Here's how the part is built. I have some questions about the finished solid (model axes, mm). A direction names the side the tool comes from. Round coordinates to 2 decimals unless told otherwise and drop trailing zeros. Write each loop counter-clockwise with the first axis right and the second up, starting at its lowest first coordinate (ties: lowest second). Pieces come first, ordered by that corner, then holes. Notation, with made-up numbers: (41, 2) -> (80, 2) arc R12 cw to (80, 16) -> close; hole circle Ø10 at (89, 87). An arc over 180 degrees is marked (long way). Answer in a Markdown table with one row per item. Add a question column.
from build123d import *

# Parameters (mm, degrees)
BOSS_EXTRU_1_DEPTH      = 23
BOSS_EXTRU_2_DEPTH      = 3
ENL_V_MAT_EXTRU_1_DEPTH = 3
ESQUISSE4_R             = 2.6
ENL_V_MAT_EXTRU_2_DEPTH = 3
ESQUISSE5_R             = 2.6
ENL_V_MAT_EXTRU_3_DEPTH = 3
ESQUISSE6_R             = 2.6
ENL_V_MAT_EXTRU_4_DEPTH = 3
CONG_1_R                = 10


with BuildPart() as part:
    # Esquisse1 → Boss.-Extru.1 (new body)
    with BuildSketch(Plane.XY):
        Polygon((100, 92.65), (100, 112.65), (97, 112.65), (97, 93.123594611), (90.984838829, 74.546771861), (93.838946748, 73.622613873), align=None)
    extrude(amount=BOSS_EXTRU_1_DEPTH)

    # Esquisse2 → Boss.-Extru.2 (add)
    with BuildSketch(Plane.XY):
        Polygon((90.984838829, 74.546771861), (79, 74.546771861), (79, 112.65), (97, 112.65), (97, 93.123594611), align=None)
    extrude(amount=BOSS_EXTRU_2_DEPTH)

    # Esquisse3 → Enlèv. mat.-Extru.1 (cut)
    with BuildSketch(Plane.XY.offset(3)):
        Polygon((90.984838829, 74.546771861), (79, 78.427453619), (79, 74.546771861), align=None)
    extrude(amount=-ENL_V_MAT_EXTRU_1_DEPTH, mode=Mode.SUBTRACT)

    # Esquisse4 → Enlèv. mat.-Extru.2 (cut)
    with BuildSketch(Plane.XY.offset(3)):
        with Locations((88, 102.65)):
            Circle(ESQUISSE4_R)
        with Locations((88, 82.65)):
            Circle(ESQUISSE4_R)
    extrude(amount=-ENL_V_MAT_EXTRU_2_DEPTH, mode=Mode.SUBTRACT)

    # Esquisse5 → Enlèv. mat.-Extru.3 (cut)
    with BuildSketch(Plane.ZY.offset(-97)):
        with Locations((13, 102.886797306)):
            Circle(ESQUISSE5_R)
    extrude(amount=-ENL_V_MAT_EXTRU_3_DEPTH, mode=Mode.SUBTRACT)

    # Esquisse6 → Enlèv. mat.-Extru.4 (cut)
    with BuildSketch(Plane(origin=(60.503141075, -19.590871368, 0), x_dir=(0, 0, 1), z_dir=(-0.9513693063481516, 0.30805266260598485, 0))):
        with Locations(Location((13, 108.712835188, 0), (0, 0, 270))):
            Circle(ESQUISSE6_R)
    extrude(amount=-ENL_V_MAT_EXTRU_4_DEPTH, mode=Mode.SUBTRACT)

    # Congé1
    cong_1_edges = [part.edges().sort_by_distance(p)[0] for p in [
        (98.5, 112.65, 23),
        (92.411892788, 74.084692867, 23),
        (79, 112.65, 1.5),
        (79, 78.427453619, 1.5),
    ]]
    fillet(cong_1_edges, radius=CONG_1_R)


solid = part.part
Item 1: If we section it at C-C on z = 8.25: Please give me the cut outline in (x, y).
Item 2: If we section it at A-A on y = 98.5: Please give me the cut outline in (x, z).
Item 3: I need wall thicknesses on line 1 along Y through (x, z) = (88, 1.85); line 2 along X through (y, z) = (99, 21); line 3 along Z through (x, y) = (81.5, 87.5). Which ranges of each line are inside material? Lowest first, please. Write a range as from..to.
Item 4: For P1, Ø10, axis at x = 90, y = 85.5, coming from the -Z side; P2, Ø12, axis at x = 86, y = 98.5, coming from the +Z side; P3, Ø1, axis at y = 94, z = 6.5, coming from the -X side; P4, Ø10, axis at y = 97.5, z = 13.5, coming from the -X side, each with a flat end and sliding along its axis, tell me the tip position at first contact or that it passes through.
Item 5: If we section it at D-D on y = 82.65: Give the number of separate pieces and of enclosed holes in the cut face, then the cut area to 3 significant figures.
Item 6: If we section it at B-B on x = 88: Please give me the cut outline in (y, z).
Item 7: If we mould it in two halves opening along Z, with no side actions, what happens to faces 1 (the flat face through (94.703, 86.029, 10.638)), 2 (the cylindrical face through (93.3, 76.8, 20)), 3 (the cylindrical face through (96.04, 85.34, 11.42)), 4 (the cylindrical face through (98.48, 101.89, 15.4))? For each: pulls with the +Z half, pulls with the -Z half, needs draft (parallel to the pull), parting line crosses it, or undercut.
Item 8: On a 3-axis mill with a long thin cutter (end or side, diameter ignored), from which of +Z, -Z, +X, -X, +Y, -Y can I reach the whole of each face in a straight line? I mean faces 5 (the flat face through (97, 100.9, 10.6)), 6 (the flat face through (97.56, 85.12, 11.34)). Say none if no direction works.
Results list:
| question | item | result |
|---|---|---|
| 1 | outline | (90.98, 74.55) -> (93.84, 73.62) -> (100, 92.65) -> (100, 112.65) -> (97, 112.65) -> (97, 93.12) -> close |
| 2 | outline | (79, 0) -> (100, 0) -> (100, 23) -> (97, 23) -> (97, 3) -> (79, 3) -> close |
| 3 | line 1 | 75.51..80.05, 85.25..100.05, 105.25..112.6 |
| 3 | line 2 | 97..100 |
| 3 | line 3 | 0..3 |
| 4 | P1 | z = 0 |
| 4 | P2 | z = 3 |
| 4 | P3 | x = 97 |
| 4 | P4 | x = 96.8 |
| 5 | separate pieces | 3 |
| 5 | enclosed holes | 0 |
| 5 | area | 83.6 mm² |
| 6 | outline | (75.51, 0) -> (80.05, 0) -> (80.05, 3) -> (75.51, 3) -> close; (85.25, 0) -> (100.05, 0) -> (100.05, 3) -> (85.25, 3) -> close; (105.25, 0) -> (112.6, 0) -> (112.6, 3) -> (105.25, 3) -> close |
| 7 | face 1 | needs draft |
| 7 | face 2 | pulls with the +Z half |
| 7 | face 3 | undercut |
| 7 | face 4 | undercut |
| 8 | face 5 | +Z, -X, +Y |
| 8 | face 6 | +Z, -Z, +X, -Y |
